Geometry: final body of the model. Coordinates: model frame, mm. A direction names the side the tool comes from. Give positions to 0.01 mm unless a question says otherwise; leave off trailing zeros. Loops run counter-clockwise (first coordinate to the right, second up) from the corner with the lowest first, then second, coordinate; pieces in that order, holes last. Notation, with made-up numbers: M -12,13.25 L 25,13.25 A16 cw 25,22.25 Z; hole C 52,-34.75 d6. An arc over 180 degrees is marked long. One line per question, with ' | ' between items. Start each with the question number.
from build123d import *

# Parameters (mm, degrees)
F1_DEPTH = 225
F3_D     = 19
F3_DEPTH = 52
F3_TIP   = 5.7081758808


with BuildPart() as f1:
    # F0 (on Front) → F1 (new body)
    with BuildSketch(Plane.XZ):
        Polygon((32.5, 21), (0, 21), (0, -23), (3, -23), (3, -29), (32.5, -29), align=None)
    extrude(amount=F1_DEPTH)

    # F3
    with Locations(Plane(origin=(0, 0, 0), x_dir=(-1, 0, 0), z_dir=(0, 1, 0))):
        with Locations((0, 0)):
            Hole(F3_D / 2, depth=F3_DEPTH)
            with Locations((0, 0, -(F3_DEPTH + F3_TIP / 2))):  # 118° drill point
                Cone(0, F3_D / 2, F3_TIP, mode=Mode.SUBTRACT)

    # F4: F1 across face


with BuildPart() as f1_1:
    add(f1.part)
    add(f1.part.mirror(Plane(origin=(0, -122.5069848753, -1.1176625039), x_dir=(0, -1, 0), z_dir=(-1, 0, 0))))


solid = f1_1.part
Q1. Section B-B, the plane y = -55. Output: boundary loops of the cut face in (x, z).
Q2. Draft query along X for faces 1 (the cylindrical face through (9.274, -26.364, -2.059)), 2 (the flat face through (32.5, -111, -4)), 3 (the flat face through (-18, -111, -29)). Return one class per face: released by +X, released by -X, zero draft, split by the parting line, or undercut.
Q3. Set-up query: faces 4 (the flat face through (0, -225, -4)), 5 (the flat face through (3, -111, -26)). Return all of +Z, -Z, +X, -X, +Y, -Y with unobstructed straight access to the full face (end or side cutting, diameter ignored); none if empty.
Q4. Section A-A, the plane z = 0. Output: boundary loops of the cut face in (x, y), plus the area to 3 significant figures.
Q5. Material intervals for L1, parallel to X at y = -30, z = 0; L2, parallel to Z at x = 0, y = -10.5; L3, parallel to X at y = -50, z = 7, sorted ascending.
Q6. Contact query for flat-ended pins moving along their axis: pin 1 (6 mm diameter, centred on x = -14, z = -17, fed in from +Y); pin 2 (15 mm diameter, centred on x = 0, z = 0, fed in from +Y); pin 3 (2.5 mm diameter, centred on x = 1, y = -100.5, fed in from -Z). Output: stop coordinate, or through.
Model answer:
1) outline: M -32.5,-29 L -3,-29 L -3,-23 L 3,-23 L 3,-29 L 32.5,-29 L 32.5,21 L -32.5,21 Z; hole C 0,0 d9.01
2) face 1: undercut | face 2: released by +X | face 3: zero draft
3) face 4: +Z, -Z, +X, -X, -Y | face 5: -Z, +Y, -Y
4) outline: M -32.5,-225 L 32.5,-225 L 32.5,0 L 9.5,0 L 9.5,-52 L 0,-57.71 L -9.5,-52 L -9.5,0 L -32.5,0 Z | area: 13,600 mm^2
5) L1: x = -32.5 to -9.5, 9.5 to 32.5 | L2: z = -23 to -9.5, 9.5 to 21 | L3: x = -32.5 to -6.42, 6.42 to 32.5
6) pin 1: stops at y = 0 | pin 2: stops at y = -53.2 | pin 3: stops at z = -23
